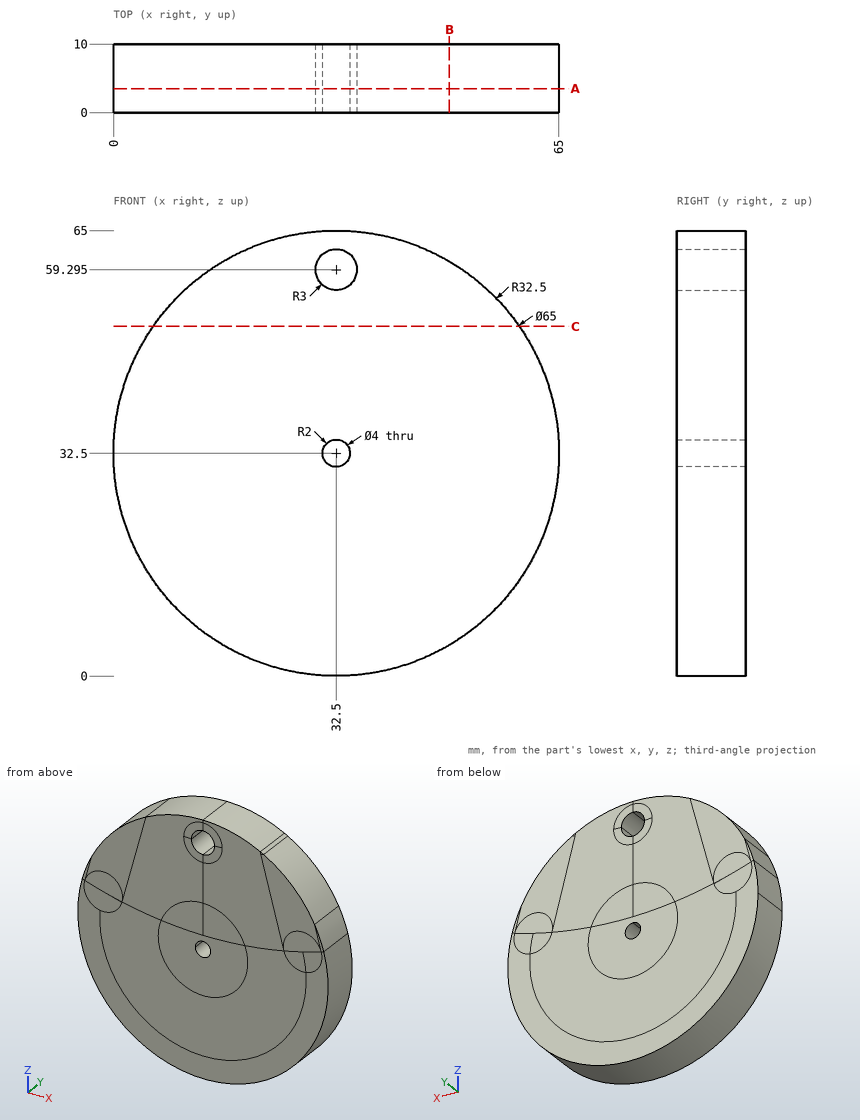
Answer from the drawing. Dimensions are ordinates in mm from the lowest x, y and z of the part. Give positions to 0.01 mm unless a question says otherwise; leave off trailing zeros. Order: outer loops, then holes, each group sorted by start corner. A loop starts at its lowest first (then second) coordinate and runs counter-clockwise, first axis right, second up. Notation, with made-up numbers: (47, 79) - (54, 79) arc R23 ccw to (54, 92) - close; hole circle Ø4 at (19.25, -26.5). An arc over 180 degrees is marked (long way). One line per item, written item: value. Start each with the question number.
1) A cutting plane is placed at C-C on z = 51. Give the vertices of the cut face in (x, y), then the cut area to 3 significant figures.
2) Given pin 1 Ø2 at (x, y) = (8.5, 1.5) entering from -Z; pin 2 Ø1 at (y, z) = (3.5, 40) entering from +X; pin 3 Ø4 at (x, y) = (35, 8) entering from -Z, each flat-ended and moving along its own axis, determine where each tip first touches the part or whether it passes through.
3) A cutting plane is placed at B-B on x = 49. Give the vertices of the cut face in (y, z).
4) A cutting plane is placed at A-A on y = 3.5. Give the vertices of the cut face in (x, z) (3 decimals), then the cut area to 3 significant figures.
5) Find the intervals of material crossed by L1, parallel to Z at x = 32.5, y = 7.5 (3 decimals); L2, parallel to X at y = 7.75, z = 32.5; L3, parallel to Z at x = 31.5, y = 4.25 (1 decimal), in increasing order.
Answer sheet:
1. outline: (5.78, 0) - (59.22, 0) - (59.22, 10) - (5.78, 10) - close
1. area: 534 mm2
2. pin 1: stops at z = 9.54
2. pin 2: stops at x = 64.24
2. pin 3: stops at z = 0
3. outline: (0, 4.5) - (10, 4.5) - (10, 60.5) - (0, 60.5) - close
4. outline: circle Ø65 at (32.5, 32.5); hole circle Ø6 at (32.5, 59.295); hole circle Ø4 at (32.5, 32.5)
4. area: 3,280 mm2
5. L1: z = 0 to 30.5, 34.5 to 56.295, 62.295 to 65
5. L2: x = 0 to 30.5, 34.5 to 65
5. L3: z = 0 to 30.8, 34.2 to 56.5, 62.1 to 65
